Check sheet for the modelled part. Datum: model origin and axes. Units: mm. A direction names the side the tool comes from. Coordinates: 2 decimals unless noted, no trailing zeros. Loops run counter-clockwise (first coordinate to the right, second up) from the corner with the lowest first, then second, coordinate; pieces in that order, holes last. Notation, with made-up numbers: (-35, 65.5) - (-22, 65.5) arc R15 cw to (-22, 71.5) - close; hole circle Ø1 at (21, -22.5). An arc over 180 degrees is marked (long way). Use a Markdown table: item, result. Add a question column.
1) Thickness scan on line 1 (Z direction, x = 0, y = -14.75); line 2 (Y direction, x = -0.3, z = 0.25); line 3 (X direction, y = 20, z = 1.85). Record the ranges inside material, lowest first.
2) Sectioned sample at C-C, the plane y = -16. Enter the section's corners in (x, z).
3) Go/stop test with flat-tipped pins: P1, Ø2, axis at x = 0, z = 0, coming from the +Y side; P2, Ø1.5, axis at y = -1.5, z = -1, coming from the -X side; P3, Ø2, axis at x = -0.5, z = 0, coming from the +Y side. Record where each tip stops, or that it passes through.
4) Sectioned sample at B-B, the plane z = 0. Enter the section's corners in (x, y), then the cut area to 3 significant figures.
5) Tool access check on faces 5 (the flat face through (-2, 22.5, 0)), 6 (the flat face through (0, 12.5, 0)), 7 (the cylindrical face through (0.748, -17.198, 0.976)). Record the directions out of +Z, -Z, +X, -X, +Y, -Y that give a thin tool (end or side, any length) a straight path to the whole face; none if there is none.
6) Draft check along X on faces 1 (the cylindrical face through (3, 0, 0)), 2 (the flat face through (-2, -22.5, 0)), 3 (the cylindrical face through (0.748, 17.198, -0.976)), 4 (the flat face through (0, -12.5, 0)). Enter one of: pulls with the +X half, pulls with the -X half, needs draft (parallel to the pull), parting line crosses it, or undercut.
7) Sectioned sample at D-D, the plane y = -11. Enter the section's corners in (x, z).
8) Sectioned sample at A-A, the plane x = 0. Enter the section's corners in (y, z).
Autodesk Inventor part; units mm, degrees
ref_plane "YZ Plane" through (0, 0, 0) normal (1, 0, 0) x (0, 1, 0)
ref_plane "XZ Plane" through (0, 0, 0) normal (0, 1, 0) x (-1, 0, 0)
ref_plane "XY Plane" through (0, 0, 0) normal (0, 0, 1) x (1, 0, 0)
sketch "スケッチ1" plane through (0, 0, 0) normal (0, 1, 0) x (-1, 0, 0)
  circle A0 centre (0, 0) radius 3
  dimension "d0" = 6
extrude "押し出し1" add sketch "スケッチ1" along normal mid plane 45
sketch "スケッチ2" plane through (0, 22.5, 0) normal (0, 1, 0) x (1, 0, 0)
  point P0 (0, 0)
  point P1 (0, 0)
hole "穴1" at (0, 22.5, 0) direction (0, -1, 0) diameter 2.459 depth 10 countersink diameter 3.4 countersink angle 90
sketch "スケッチ3" plane through (0, -22.5, 0) normal (0, -1, 0) x (1, 0, 0)
  point P0 (0, 0)
  point P1 (0, 0)
hole "穴2" at (0, -22.5, 0) direction (0, 1, 0) diameter 2.459 depth 10 countersink diameter 3.4 countersink angle 90
chamfer "面取り1" distance 0.25 angle 45 2 edges at (3, -22.5, 0) (3, 22.5, 0)
properties part number "Spacer_M3D6L45" material "アルミニウム 6061"
Solved:
| question | item | result |
|---|---|---|
| 1 | line 1 | z = -3 to -1.23, 1.23 to 3 |
| 1 | line 2 | y = -12.5 to 12.5 |
| 1 | line 3 | x = -2.36 to 2.36 |
| 2 | outline | circle Ø6 at (0, 0); hole circle Ø2.46 at (0, 0) |
| 3 | P1 | stops at y = 12.5 |
| 3 | P2 | stops at x = -2.99 |
| 3 | P3 | stops at y = 22.3 |
| 4 | outline | (-3, -22.25) - (-2.75, -22.5) - (-1.7, -22.5) - (-1.23, -22.03) - (-1.23, -12.5) - (1.23, -12.5) - (1.23, -22.03) - (1.7, -22.5) - (2.75, -22.5) - (3, -22.25) - (3, 22.25) - (2.75, 22.5) - (1.7, 22.5) - (1.23, 22.03) - (1.23, 12.5) - (-1.23, 12.5) - (-1.23, 22.03) - (-1.7, 22.5) - (-2.75, 22.5) - (-3, 22.25) - close |
| 4 | area | 220 mm2 |
| 5 | face 5 | +Z, -Z, +X, -X, +Y |
| 5 | face 6 | +Y |
| 5 | face 7 | -Y |
| 6 | face 1 | parting line crosses it |
| 6 | face 2 | needs draft |
| 6 | face 3 | undercut |
| 6 | face 4 | undercut |
| 7 | outline | circle Ø6 at (0, 0) |
| 8 | outline | (-22.5, -2.75) - (-22.25, -3) - (22.25, -3) - (22.5, -2.75) - (22.5, -1.7) - (22.03, -1.23) - (12.5, -1.23) - (12.5, 1.23) - (22.03, 1.23) - (22.5, 1.7) - (22.5, 2.75) - (22.25, 3) - (-22.25, 3) - (-22.5, 2.75) - (-22.5, 1.7) - (-22.03, 1.23) - (-12.5, 1.23) - (-12.5, -1.23) - (-22.03, -1.23) - (-22.5, -1.7) - close |
